```python
from build123d import *

# Parameters (mm, degrees)
SKETCH2_W           = 42.418
SKETCH2_H           = 20.32
BOSS_EXTRUDE1_DEPTH = 12.319
SKETCH5_W           = 12.7
SKETCH5_H           = 20.32
CUT_EXTRUDE1_DEPTH  = 9.779
SKETCH6_W           = 12.7
SKETCH6_H           = 20.32
CUT_EXTRUDE2_DEPTH  = 9.779
SKETCH7_W           = 11.938
SKETCH7_H           = 20.32
CUT_EXTRUDE3_DEPTH  = 9.779
SKETCH8_R           = 2.54
CUT_EXTRUDE4_DEPTH  = 2.54
SKETCH9_R           = 2.54
CUT_EXTRUDE5_DEPTH  = 2.54


with BuildPart() as part:
    # Sketch2 → Boss-Extrude1 (new body)
    with BuildSketch(Plane(origin=(0, 0, 0), x_dir=(1, 0, 0), z_dir=(0, 1, 0))):
        with Locations((15.610403741, -5.358242937)):
            Rectangle(SKETCH2_W, SKETCH2_H)
    extrude(amount=BOSS_EXTRUDE1_DEPTH)

    # Sketch5 → Cut-Extrude1 (cut)
    with BuildSketch(Plane(origin=(0, 12.319, 0), x_dir=(1, 0, 0), z_dir=(0, 1, 0))):
        with Locations((0.751403741, -5.358242937)):
            Rectangle(SKETCH5_W, SKETCH5_H)
    extrude(amount=-CUT_EXTRUDE1_DEPTH, mode=Mode.SUBTRACT)

    # Sketch6 → Cut-Extrude2 (cut)
    with BuildSketch(Plane(origin=(0, 12.319, 0), x_dir=(1, 0, 0), z_dir=(0, 1, 0))):
        with Locations((30.469403741, -5.358242937)):
            Rectangle(SKETCH6_W, SKETCH6_H)
    extrude(amount=-CUT_EXTRUDE2_DEPTH, mode=Mode.SUBTRACT)

    # Sketch7 → Cut-Extrude3 (cut)
    with BuildSketch(Plane(origin=(0, 0, 0), x_dir=(-1, 0, 0), z_dir=(0, -1, 0))):
        with Locations((-15.610403741, -5.358242937)):
            Rectangle(SKETCH7_W, SKETCH7_H)
    extrude(amount=-CUT_EXTRUDE3_DEPTH, mode=Mode.SUBTRACT)

    # Sketch8 → Cut-Extrude4 (cut)
    with BuildSketch(Plane(origin=(0, 2.54, 0), x_dir=(1, 0, 0), z_dir=(0, 1, 0))):
        with Locations(Location((0.751403741, -5.358242937, 0), (0, 0, 270))):
            Circle(SKETCH8_R)
    extrude(amount=-CUT_EXTRUDE4_DEPTH, mode=Mode.SUBTRACT)

    # Sketch9 → Cut-Extrude5 (cut)
    with BuildSketch(Plane(origin=(0, 2.54, 0), x_dir=(1, 0, 0), z_dir=(0, 1, 0))):
        with Locations(Location((30.469403741, -5.358242937, 0), (0, 0, 270))):
            Circle(SKETCH9_R)
    extrude(amount=-CUT_EXTRUDE5_DEPTH, mode=Mode.SUBTRACT)


solid = part.part
```
Input: part model. Units: mm. Frame: model coordinates. A direction names the side the tool comes from. Give positions to 0.01 mm unless a question says otherwise; leave off trailing zeros. Loops run counter-clockwise (first coordinate to the right, second up) from the corner with the lowest first, then second, coordinate; pieces in that order, holes last. Notation, with made-up numbers: (34.25, 56.25) -> (55.25, 56.25) arc R26 ccw to (55.25, 78.25) -> close; hole circle Ø3 at (86.25, 62). An arc over 180 degrees is marked (long way). Use a Markdown table: item, result.
Q1. Access query for faces 4 (the flat face through (-1, 2.54, 3)), 5 (the flat face through (29, 2.54, 3)), 6 (the flat face through (16, 9.779, 5)), 7 (the flat face through (14, 10, -4.802)). Directions: +Z, -Z, +X, -X, +Y, -Y. A direction counts if a zero-diameter tool reaches every point of the face in a straight line with its end or side. Return the directions, or none.
Entries:
| item | result |
|---|---|
| face 4 | +Z, -Z, -X, +Y |
| face 5 | +Z, -Z, +X, +Y |
| face 6 | +Z, -Z, -Y |
| face 7 | -Z, +X, -X, +Y, -Y |
Q2. Pull-direction query (X, two-part tool) for faces 1 (the flat face through (36.819, 1, 6)), 2 (the flat face through (15, 12.319, 5)), 3 (the cylindrical face through (32.99, 1.29, 5.03)); classes: pulls with the +X half, pulls with the -X half, needs draft (parallel to the pull), parting line crosses it, or undercut.
Entries:
| item | result |
|---|---|
| face 1 | pulls with the +X half |
| face 2 | needs draft |
| face 3 | undercut |
Q3. Section query D-D, the plane x = 2.5. Return the cut outline in (y, z).
Entries:
| item | result |
|---|---|
| outline | (0, -4.8) -> (2.54, -4.8) -> (2.54, 3.52) -> (0, 3.52) -> close; (0, 7.2) -> (2.54, 7.2) -> (2.54, 15.52) -> (0, 15.52) -> close |
Q4. First-contact query: P1, Ø6.5, axis at x = 27.5, z = 3.5, coming from the +Y side; P2, Ø6, axis at x = 17, z = 5.5, coming from the -Y side; P3, Ø1.5, axis at y = 7.5, z = 3.5, coming from the -X side; P4, Ø3, axis at x = 30.47, z = 5.36, coming from the -Y side. Flat tips, straight axial feed; report the tip coordinate or a pass-through.
Entries:
| item | result |
|---|---|
| P1 | stops at y = 2.54 |
| P2 | stops at y = 9.78 |
| P3 | stops at x = 7.1 |
| P4 | passes through |
Q5. Ray query, probe 1 along X at (y, z) = (0.75, -0.5); probe 2 along X at (y, z) = (8, 10.5); probe 3 along Y at (x, z) = (0, -0.75). Return the intervals inside material, ascending. Write a range as from..to.
Entries:
| item | result |
|---|---|
| probe 1 | x = -5.6..9.64, 21.58..36.82 |
| probe 2 | x = 7.1..9.64, 21.58..24.12 |
| probe 3 | y = 0..2.54 |
Q6. Section query B-B, the plane z = 0. Return the cut outline in (x, y).
Entries:
| item | result |
|---|---|
| outline | (-5.6, 0) -> (9.64, 0) -> (9.64, 9.78) -> (21.58, 9.78) -> (21.58, 0) -> (36.82, 0) -> (36.82, 2.54) -> (24.12, 2.54) -> (24.12, 12.32) -> (7.1, 12.32) -> (7.1, 2.54) -> (-5.6, 2.54) -> close |
Q7. Section query C-C, the plane z = 5. Return the cut outline in (x, y), plus the area to 3 significant figures.
Entries:
| item | result |
|---|---|
| outline | (-5.6, 0) -> (-1.76, 0) -> (-1.76, 2.54) -> (-5.6, 2.54) -> close; (3.27, 0) -> (9.64, 0) -> (9.64, 9.78) -> (21.58, 9.78) -> (21.58, 0) -> (27.95, 0) -> (27.95, 2.54) -> (24.12, 2.54) -> (24.12, 12.32) -> (7.1, 12.32) -> (7.1, 2.54) -> (3.27, 2.54) -> close; (32.98, 0) -> (36.82, 0) -> (36.82, 2.54) -> (32.98, 2.54) -> close |
| area | 132 mm² |
Q8. Section query A-A, the plane y = 7. Return the cut outline in (x, z).
Entries:
| item | result |
|---|---|
| outline | (7.1, -4.8) -> (9.64, -4.8) -> (9.64, 15.52) -> (7.1, 15.52) -> close; (21.58, -4.8) -> (24.12, -4.8) -> (24.12, 15.52) -> (21.58, 15.52) -> close |
